Design review of the part built by this model. Coordinates are the model's own, in mm. Face numbers are marked on the shaded views. Round coordinates to 2 decimals unless told otherwise and drop trailing zeros. Loops run counter-clockwise (first coordinate to the right, second up) from the corner with the lowest first, then second, coordinate; pieces in that order, holes last. Notation, with made-up numbers: (66, 38) -> (105, 38) arc R31 ccw to (105, 74) -> close; hole circle Ø7 at (55, 21.25). An arc over 180 degrees is marked (long way). Answer as CSV lines item,"result". Start each with the question number.
Autodesk Inventor part; units mm, degrees
ref_plane "Work Plane1" through (59.9208, 47.0911, 21.911) normal (0, 1, 0) x (-1, 0, 0)
ref_plane "Work Plane2" through (59.9208, 45.8611, 21.911) normal (0, -1, 0) x (1, 0, 0)
ref_plane "Work Plane13" through (59.9208, 43.8611, -18.7491) normal (1, 0, 0) x (0, 0, -1)
ref_plane "Work Plane1" through (59.9208, 47.0911, 21.911) normal (0, 1, 0) x (-1, 0, 0)
sketch "Sketch1" plane through (59.9208, 47.0911, 21.911) normal (0, 1, 0) x (-1, 0, 0)
  circle A0 centre (-16.808, -43.6345) radius 1.27
  circle A1 centre (12.5729, -47.6345) radius 1.27
  circle A2 centre (16.4459, -43.6345) radius 1.27
  circle A3 centre (-12.808, -47.6345) radius 1.27
  line L0 (10.208, -33.8805) -> (10.208, -44.6601)
  line L1 (10.208, -44.6601) -> (6.6725, -48.1956)
  circle A4 centre (-16.808, -43.6345) radius 1.27
  circle A5 centre (12.5729, -47.6345) radius 1.27
  circle A6 centre (16.4459, -43.6345) radius 1.27
  circle A7 centre (-12.8081, -47.6345) radius 1.27
  line L2 (19.708, -15.6655) -> (-19.708, -15.6655)
  line L3 (0, -15.6655) -> (0, -20.8781)
  line L4 (6.6725, -48.1956) -> (-7.3796, -48.1956)
  line L5 (-19.958, -43.8381) -> (-12.8316, -50.9645)
  line L6 (-12.8316, -50.9645) -> (12.8316, -50.9645)
  line L7 (-19.958, -40.6601) -> (-19.958, -43.8381)
  line L8 (0, -48.1956) -> (0, -46.7038)
  line L9 (19.958, -43.8381) -> (12.8316, -50.9645)
  line L10 (19.958, -40.6601) -> (19.958, -43.8381)
  line L11 (-11.938, -30.6601) -> (-11.938, -43.6372)
  line L12 (-10.5616, -45.0137) -> (-11.938, -43.6372)
  line L13 (-10.5616, -45.0137) -> (-7.3796, -48.1956)
  line L14 (15.2967, -30.6601) -> (18.458, -30.6601)
  line L15 (18.458, -30.6601) -> (18.458, -39.1601)
  line L16 (-18.458, -39.1601) -> (-18.458, -30.6601)
  line L17 (-18.458, -30.6601) -> (-11.938, -30.6601)
  line L18 (10.208, -33.8805) -> (15.2967, -33.8805)
  line L19 (15.2967, -33.8805) -> (15.2967, -30.6601)
  line L20 (-19.958, -40.6601) -> (-18.458, -39.1601)
  line L21 (19.958, -40.6601) -> (18.458, -39.1601)
  point P0 (-19.708, -43.6601)
  point P1 (-6.6725, -48.1956)
  dimension "d14" = 5
  dimension "d15" = 135
  dimension "d18" = 2.54
extrude "Extrusion1" add sketch "Sketch1" along normal blind 2
ref_plane "Work Plane2" through (59.9208, 45.8611, 21.911) normal (0, -1, 0) x (1, 0, 0)
sketch "Sketch2" plane through (59.9208, 45.8611, 21.911) normal (0, -1, 0) x (1, 0, 0)
  line L0 (-10.208, -33.8805) -> (-10.208, -44.6601)
  line L1 (-10.208, -44.6601) -> (-6.6725, -48.1956)
  line L2 (-6.6725, -48.1956) -> (7.3796, -48.1956)
  circle A0 centre (16.808, -43.6345) radius 1.27
  circle A1 centre (-12.5729, -47.6345) radius 1.27
  circle A2 centre (-16.4459, -43.6345) radius 1.27
  circle A3 centre (12.808, -47.6345) radius 1.27
  line L3 (19.958, -40.6601) -> (19.958, -43.8381)
  line L4 (19.958, -43.8381) -> (12.8316, -50.9645)
  line L5 (12.8316, -50.9645) -> (-12.8316, -50.9645)
  line L6 (-12.8316, -50.9645) -> (-19.958, -43.8381)
  line L7 (-19.958, -43.8381) -> (-19.958, -40.6601)
  line L8 (7.3796, -48.1956) -> (11.938, -43.6372)
  line L9 (11.938, -43.6372) -> (11.938, -30.6601)
  line L10 (11.938, -30.6601) -> (18.458, -30.6601)
  line L11 (18.458, -30.6601) -> (18.458, -39.1601)
  line L12 (-18.458, -39.1601) -> (-18.458, -30.6601)
  line L13 (-18.458, -30.6601) -> (-15.2967, -30.6601)
  line L14 (-15.2967, -30.6601) -> (-15.2967, -33.8805)
  line L15 (-15.2967, -33.8805) -> (-10.208, -33.8805)
  line L16 (18.458, -39.1601) -> (19.958, -40.6601)
  line L17 (-19.958, -40.6601) -> (-18.458, -39.1601)
  circle A4 centre (-16.4459, -43.6345) radius 1.27
  line L18 (-19.958, -43.8381) -> (-19.958, -40.6601)
  line L19 (-19.958, -41.5123) -> (-10.208, -41.5123)
  line L20 (-10.208, -33.8805) -> (-10.208, -44.6601)
  point P0 (-59.9208, -21.911)
extrude "Extrusion2" add sketch "Sketch2" along normal blind 2 contours L0 L1 L2 L8 L9 L10 L11 L16 L3 L4 L5 L6 L7 L19
sketch "Sketch4" plane through (79.8789, 45.8611, -18.7491) normal (1, 0, 0) x (0, 0, -1)
  line L0 (0, 1.23) -> (3.178, 1.23)
  line L1 (0, 0) -> (-1.5, 0)
  line L2 (0, 1.23) -> (0, 0)
  line L3 (-12.1065, -0.085) -> (12.1065, -0.085)
  line L4 (12.1065, -0.085) -> (12.1065, 1.315)
  line L5 (12.1065, 1.315) -> (-12.1065, 1.315)
  line L6 (-12.1065, 1.315) -> (-12.1065, -0.085)
  line L7 (-12.1065, -0.085) -> (12.1065, 1.315) construction
  line L8 (12.1065, -0.085) -> (-12.1065, 1.315) construction
  point P0 (0, 0.615)
  dimension "d73" = 1.4
extrude "Extrusion3" cut sketch "Sketch4" against normal through all
sketch "Sketch5" plane through (59.9208, 43.8611, 21.911) normal (0, -1, 0) x (1, 0, 0)
  line L0 (-19.708, -43.6601) -> (-19.708, -40.6601)
  line L1 (-12.6424, -50.7145) -> (-19.708, -43.6601)
  line L2 (12.728, -50.7145) -> (-12.6424, -50.7145)
  line L3 (19.708, -43.7345) -> (12.728, -50.7145)
  line L4 (-13.4529, -52.4645) -> (13.4529, -52.4645)
  line L5 (19.708, -43.7345) -> (19.708, -40.6601)
  line L6 (-12.8316, -50.9145) -> (12.8316, -50.9145)
  line L7 (12.8316, -50.9645) -> (11.3316, -52.4645)
  line L8 (-19.958, -43.8381) -> (-12.8316, -50.9645)
  line L9 (-12.8316, -50.9645) -> (-11.3316, -52.4645)
  line L10 (-12.8316, -50.9645) -> (-10.7103, -50.9645) construction
  line L11 (12.8316, -50.9145) -> (12.8816, -50.9145)
  line L12 (-12.8316, -50.9645) -> (12.8316, -50.9645)
  line L13 (12.8316, -50.9645) -> (12.8816, -50.9145)
  line L14 (12.8316, -50.9645) -> (19.958, -43.8381)
  line L15 (-12.8316, -50.9145) -> (-12.8816, -50.9145)
  line L16 (-12.8316, -50.9645) -> (-12.8816, -50.9145)
  line L17 (12.8109, -50.9145) -> (19.958, -43.7673)
  line L18 (-19.958, -43.7673) -> (-12.8109, -50.9145)
  line L19 (-19.958, -45.9594) -> (-13.4529, -52.4645)
  line L20 (13.4529, -52.4645) -> (19.958, -45.9594)
  line L21 (-19.958, -43.7673) -> (-19.958, -45.9594)
  line L22 (12.8316, -50.9645) -> (19.958, -43.8381)
  line L23 (19.958, -43.8381) -> (19.958, -45.9594)
  line L24 (19.958, -43.8381) -> (19.958, -43.7673)
  line L25 (19.958, -43.8381) -> (19.958, -40.6601)
  dimension "d29" = 0.2
  dimension "d62" = 45
  dimension "d74" = 0.05
  dimension "d75" = 0.05
  dimension "d76" = 1.5
  dimension "d77" = 1.5
extrude "Extrusion4" add sketch "Sketch5" against normal up to surface (5.23 mm away)
ref_plane "Work Plane13" through (59.9208, 43.8611, -18.7491) normal (1, 0, 0) x (0, 0, -1)
ref_plane "Work Plane14" through (53.2483, 46.4761, -26.2847) normal (0, 1, 0) x (1, 0, 0)
sketch "Sketch18" plane through (59.9208, 43.8611, -18.7491) normal (1, 0, 0) x (0, 0, -1)
  line L0 (11.8044, 0) -> (10.0544, 0)
  line L1 (10.0544, 0) -> (10.0544, -2)
  line L2 (10.0544, -2) -> (11.8044, -0.5316)
  line L3 (11.8044, -0.5316) -> (11.8044, 0)
  line L4 (14.6328, 1.8418) -> (14.6328, 3.6226)
  line L5 (14.2086, 3.6226) -> (13.2186, 2.6326)
  line L6 (13.2186, 2.6326) -> (12.3544, 2.6326)
  line L7 (11.8044, 3.1826) -> (11.8044, 0)
  line L8 (11.8044, -0.5316) -> (14.6328, 1.8418)
  line L9 (11.8044, -0.5316) -> (15.8044, -0.5316) construction
  line L10 (14.2086, 3.6226) -> (14.6328, 3.6226)
  line L11 (11.9924, 3.2605) -> (12.4323, 2.8206)
  line L12 (11.8044, 3.1826) -> (12.3544, 2.6326)
  dimension "d184" = 1.75
  dimension "d185" = 2
  dimension "d186" = 50
  dimension "d198" = 135
  dimension "d203" = 40
extrude "Extrusion12" add sketch "Sketch18" along normal blind 8.804 and the other way blind 8.804
properties part number "Button Holder"
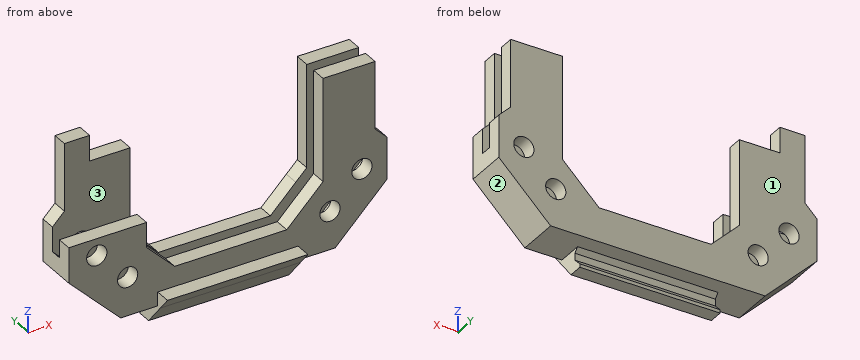
Q1. Add section D-D, the plane z = -28. Give the boundary of the cut face in (x, y), and give its area (3 significant figures).
Q2. For pin 1 Ø1.5 at (y, z) = (48.5, -13.5) entering from +X; pin 2 Ø4 at (x, y) = (47.5, 47) entering from +Z; pin 3 Ø10 at (x, z) = (65.5, -17) entering from -Y; pin 4 Ø3.5 at (y, z) = (44, -31.5) entering from -X, all flat-tipped, find the tip position at first contact; note any pin that passes through.
Q3. Mouldability with a two-part tool opening along Y and no side actions: class the marked faces 1, 2 and 3 as pulls with the +Y half, pulls with the -Y half, needs draft (parallel to the pull), parting line crosses it, or undercut.
Q4. Add section B-B, the plane x = 77.5. Give the boundary of the cut face in (y, z), and give its area (3 significant figures).
Q5. Add section A-A, the plane z = -11. Give the boundary of the cut face in (x, y).
Q6. Add section C-C, the plane y = 48.5. Give the boundary of the cut face in (x, z), and give its area (3 significant figures).
Q7. To check wall thickness, follow probe 1 along Y at (x, z) = (72, -14); probe 2 along X at (y, z) = (47.25, -12.75); probe 3 along Y at (x, z) = (48, -18.5). State the ranges of each line that lie inside material, in increasing order. Write a range as from..to.
Worked answers:
1,outline,"(43.91, 43.86) -> (75.93, 43.86) -> (75.93, 49.09) -> (43.91, 49.09) -> close; hole (46.11, 45.78) -> (73.74, 45.78) -> (73.74, 47.18) -> (46.11, 47.18) -> close"
1,area,"129 mm^2"
2,pin 1,"stops at x = 78.38"
2,pin 2,"stops at z = -11.97"
2,pin 3,"passes through"
2,pin 4,"stops at x = 45.66"
3,face 1,"pulls with the +Y half"
3,face 2,"needs draft"
3,face 3,"undercut"
4,outline,"(43.86, -26.43) -> (49.09, -26.43) -> (49.09, -22.73) -> (47.18, -22.73) -> (47.18, -24.24) -> (45.78, -24.24) -> (45.78, -22.73) -> (43.86, -22.73) -> close; (43.86, -20.71) -> (45.78, -20.71) -> (45.78, -8.75) -> (43.86, -8.75) -> close; (47.18, -20.71) -> (49.09, -20.71) -> (49.09, -8.75) -> (47.18, -8.75) -> close"
4,area,"63.0 mm^2"
5,outline,"(41.46, 47.18) -> (44.62, 47.18) -> (44.62, 49.09) -> (41.46, 49.09) -> close; (71.86, 43.86) -> (78.38, 43.86) -> (78.38, 45.78) -> (71.86, 45.78) -> close; (71.86, 47.18) -> (78.38, 47.18) -> (78.38, 49.09) -> (71.86, 49.09) -> close"
6,outline,"(39.96, -24.05) -> (46.47, -30.55) -> (73.37, -30.55) -> (79.88, -24.05) -> (79.88, -18.75) -> (78.38, -17.25) -> (78.38, -8.75) -> (71.86, -8.75) -> (71.86, -21.73) -> (70.48, -23.1) -> (67.3, -26.28) -> (53.25, -26.28) -> (49.71, -22.75) -> (49.71, -11.97) -> (44.62, -11.97) -> (44.62, -8.75) -> (41.46, -8.75) -> (41.46, -17.25) -> (39.96, -18.75) -> close; hole circle Ø2.54 at (43.47, -21.72); hole circle Ø2.54 at (47.35, -25.72); hole circle Ø2.54 at (72.73, -25.72); hole circle Ø2.54 at (76.73, -21.72)"
6,area,"392 mm^2"
7,probe 1,"y = 43.86..45.78, 47.18..49.09"
7,probe 2,"x = 41.46..49.71, 71.86..78.38"
7,probe 3,"y = 47.18..49.09"
